Drawing for the job (mm, zero at the part's lowest x, y, z). Coordinates: 2 decimals unless noted, no trailing zeros. Write each loop counter-clockwise with the first axis right and the second up, starting at its lowest first coordinate (ties: lowest second). Pieces come first, ordered by that corner, then holes. Notation, with made-up numbers: M 47,-17.75 L 95,-17.75 A22 ccw 95,13.25 Z; hole C 39,2 d8. An arc over 180 degrees is marked long. Use a Markdown table: item, result. Add a question column.
Q1. Slice it at C-C on z = 5. Write the cut outline in (x, y) (3 decimals), then the cut area to 3 significant figures.
Q2. Slice it at A-A on x = 56.25. Write the cut outline in (y, z) (3 decimals), then the cut area to 3 significant figures.
Q3. Slice it at D-D on x = 26.5. Write the cut outline in (y, z).
Q4. Mould opens along X. For the marked faces 1, 2 and 3 say: released by +X, released by -X, zero draft, split by the parting line, or undercut.
Q5. Wall check: L1, parallel to X at y = 0.55, z = 5 (3 decimals); L2, parallel to X at y = 4.5, z = 5 (3 decimals); L3, parallel to Y at x = 39, z = 5.75. Give the ranges that are in metal, low to high. Write a range as from..to.
Q6. Pin check, flat tips, straight feed: pin 1 Ø3 at (x, z) = (56.25, 5) entering from +Y; pin 2 Ø1.5 at (x, z) = (33, 1) entering from +Y. Stop position of each tip, or through.
Q7. Slice it at B-B on y = 3.25. Write the cut outline in (x, z) (3 decimals).
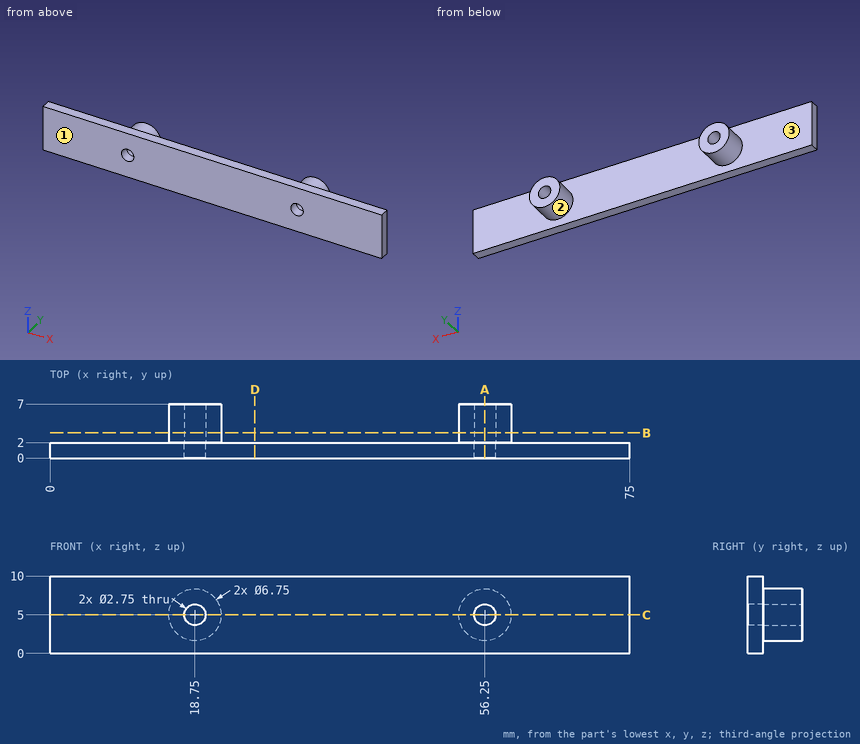
Recorded:
| question | item | result |
|---|---|---|
| 1 | outline | M 0,0 L 17.375,0 L 17.375,7 L 15.375,7 L 15.375,2 L 0,2 Z; M 20.125,0 L 54.875,0 L 54.875,7 L 52.875,7 L 52.875,2 L 22.125,2 L 22.125,7 L 20.125,7 Z; M 57.625,0 L 75,0 L 75,2 L 59.625,2 L 59.625,7 L 57.625,7 Z |
| 1 | area | 179 mm² |
| 2 | outline | M 0,0 L 2,0 L 2,1.625 L 7,1.625 L 7,3.625 L 0,3.625 Z; M 0,6.375 L 7,6.375 L 7,8.375 L 2,8.375 L 2,10 L 0,10 Z |
| 2 | area | 34.5 mm² |
| 3 | outline | M 0,0 L 2,0 L 2,10 L 0,10 Z |
| 4 | face 1 | zero draft |
| 4 | face 2 | undercut |
| 4 | face 3 | undercut |
| 5 | L1 | 0..17.375, 20.125..54.875, 57.625..75 |
| 5 | L2 | 15.375..17.375, 20.125..22.125, 52.875..54.875, 57.625..59.625 |
| 5 | L3 | 0..2 |
| 6 | pin 1 | y = 7 |
| 6 | pin 2 | y = 2 |
| 7 | outline | C 18.75,5 d6.75; C 56.25,5 d6.75; hole C 18.75,5 d2.75; hole C 56.25,5 d2.75 |
